Verification items for this drawing (mm, ordinates from the low corner). Round coordinates to 2 decimals unless told otherwise and drop trailing zeros. Write each loop counter-clockwise with the first axis right and the second up, starting at its lowest first coordinate (ties: lowest second). Pieces come first, ordered by that corner, then holes. Notation, with made-up numbers: (17, 23) -> (29, 23) arc R26 ccw to (29, 48) -> close; hole circle Ø7 at (52, 62). An arc over 180 degrees is marked (long way). Return JSON: item names as keys, results as strings. Group by question number.
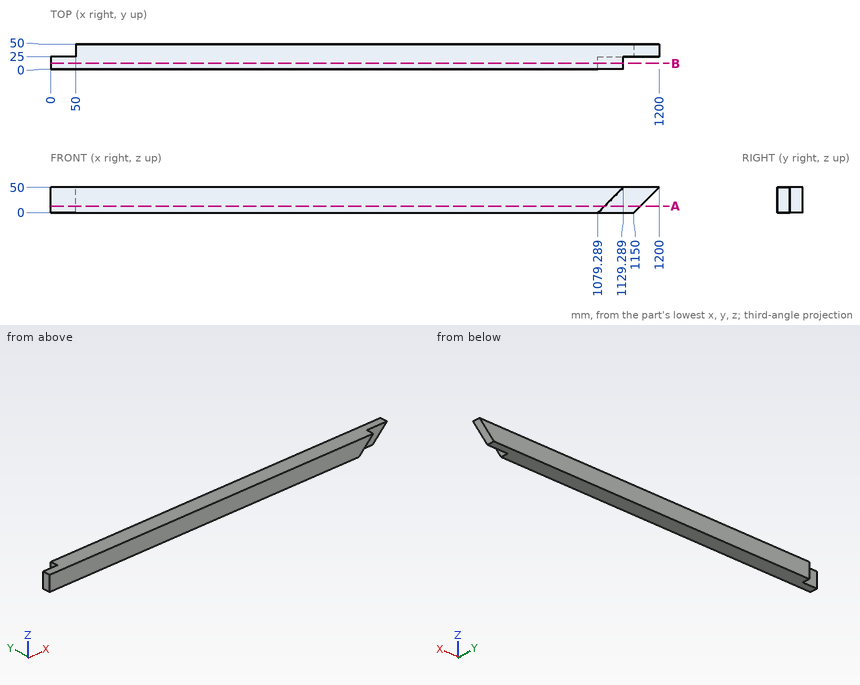
1) Go/stop test with flat-tipped pins: P1, Ø12, axis at y = 14.5, z = 18, coming from the +X side; P2, Ø12, axis at y = 28, z = 39.5, coming from the -X side; P3, Ø10, axis at y = 43.5, z = 32.5, coming from the -X side; P4, Ø15, axis at x = 1132, z = 36.5, coming from the -Y side. Record where each tip stops, or that it passes through.
2) Sectioned sample at B-B on y = 12. Enter the section's corners in (x, z).
3) Material ranges on probe 1 along X at (y, z) = (47.5, 47.5); probe 2 along X at (y, z) = (4.5, 18), recorded low to high. Write a range as [from, to].
4) Sectioned sample at A-A on z = 13. Enter the section's corners in (x, y), and give its area (3 significant figures).
Evaluation:
{
 "1": {"P1": "stops at x = 1103.29", "P2": "stops at x = 0", "P3": "stops at x = 50", "P4": "stops at y = 25"},
 "2": {"outline": "(0, 0) -> (1079.29, 0) -> (1129.29, 50) -> (0, 50) -> close"},
 "3": {"probe 1": "x = [50, 1197.5]", "probe 2": "x = [0, 1097.29]"},
 "4": {"outline": "(0, 0) -> (1092.29, 0) -> (1092.29, 25) -> (1163, 25) -> (1163, 50) -> (50, 50) -> (50, 25) -> (0, 25) -> close", "area": "55,100 mm2"}
}
